from build123d import *

# Parameters (mm, degrees)
F0_R     = 20.6375
F1_DEPTH = 6.35


# Not quite as in the source:
# - a feature names something its author has since deleted; it is built from what else it names


with BuildPart() as f1:
    # F0 (on Top) → F1 (new body)
    with BuildSketch(Plane.XY):
        with BuildLine():
            Line((-44.45, -9.525), (-75.6023437137, -9.525))
            ThreePointArc((-75.6023437137, -9.525), (-65.9911357684, -38.1), (-46.0500638279, -60.7110502417))
            Line((-46.0500638279, -60.7110502417), (-30.473891971, -33.7323291982))
            ThreePointArc((-30.473891971, -33.7323291982), (-17.4625, -30.2459372272), (-13.976108029, -43.2573291982))
            Line((-13.976108029, -43.2573291982), (-29.5522798858, -70.2360502417))
            ThreePointArc((-29.5522798858, -70.2360502417), (0, -76.2), (29.5522798858, -70.2360502417))
            Line((29.5522798858, -70.2360502417), (13.976108029, -43.2573291982))
            ThreePointArc((13.976108029, -43.2573291982), (17.4625, -30.2459372272), (30.473891971, -33.7323291982))
            Line((30.473891971, -33.7323291982), (46.0500638279, -60.7110502417))
            ThreePointArc((46.0500638279, -60.7110502417), (65.9911357684, -38.1), (75.6023437137, -9.525))
            Line((75.6023437137, -9.525), (44.45, -9.525))
            ThreePointArc((44.45, -9.525), (34.925, 0), (44.45, 9.525))
            Line((44.45, 9.525), (75.6023437137, 9.525))
            ThreePointArc((75.6023437137, 9.525), (65.9911357684, 38.1), (46.0500638279, 60.7110502417))
            Line((46.0500638279, 60.7110502417), (30.473891971, 33.7323291982))
            ThreePointArc((30.473891971, 33.7323291982), (17.4625, 30.2459372272), (13.976108029, 43.2573291982))
            Line((13.976108029, 43.2573291982), (29.5522798858, 70.2360502417))
            ThreePointArc((29.5522798858, 70.2360502417), (0, 76.2), (-29.5522798858, 70.2360502417))
            Line((-29.5522798858, 70.2360502417), (-13.976108029, 43.2573291982))
            ThreePointArc((-13.976108029, 43.2573291982), (-17.4625, 30.2459372272), (-30.473891971, 33.7323291982))
            Line((-30.473891971, 33.7323291982), (-46.0500638279, 60.7110502417))
            ThreePointArc((-46.0500638279, 60.7110502417), (-65.9911357684, 38.1), (-75.6023437137, 9.525))
            Line((-75.6023437137, 9.525), (-44.45, 9.525))
            ThreePointArc((-44.45, 9.525), (-34.925, 0), (-44.45, -9.525))
        make_face()
        Circle(F0_R, mode=Mode.SUBTRACT)
    extrude(amount=F1_DEPTH)


solid = f1.part
Geometry: final body of the model. Coordinates: model frame, mm. A direction names the side the tool comes from. Give positions to 0.01 mm unless a question says otherwise; leave off trailing zeros. Loops run counter-clockwise (first coordinate to the right, second up) from the corner with the lowest first, then second, coordinate; pieces in that order, holes last. Notation, with made-up numbers: (-3, -30) - (30, -30) arc R29 cw to (30, 8) - close; hole circle Ø8 at (-29.75, 33.25). An arc over 180 degrees is marked (long way). One line per question, with ' | ' between items. Start each with the question number.
(1) Reachability of faces 1 (the flat face through (38.37, 47.41, 3.13)), 2 (the flat face through (21.655, 56.558, 3.131)), 3 (the flat face through (60, -9.525, 3)), 4 (the flat face through (-60, 9.525, 3)) from +Z, -Z, +X, -X, +Y, -Y: full face, straight path, thin tool, end or side. Return the list, or none.
(2) Section query B-B on x = 0. Return loops of the section in (y, z).
(3) Ray query, line 1 (X direction, y = -55, z = 1.5); line 2 (Y direction, x = 0, z = 4.5); line 3 (X direction, y = -46, z = 4.25). Return the intervals inside material, ascending. Write a range as from..to.
(4) Pull-direction query (X, two-part tool) for faces 5 (the cylindrical face through (-0.4, -76.2, 3.1)), 6 (the flat face through (60, 9.525, 3)), 7 (the flat face through (21.873, -56.936, 3.131)), 8 (the cylindrical face through (65.778, -38.467, 3.131)); classes: released by +X, released by -X, zero draft, split by the parting line, or undercut.
(5) Contact query for flat-ended pins moving along their axis: pin 1 (1 mm diameter, centred on x = -9.5, z = 5, fed in from +Y); pin 2 (1 mm diameter, centred on x = -40.5, z = 1, fed in from +Y); pin 3 (3 mm diameter, centred on x = -63.5, z = 1.5, fed in from +Y). Output: stop coordinate, or through.
(6) Section query D-D on x = 33. Return loops of the section in (y, z).
The answers:
1) face 1: +Z, -Z, +Y | face 2: +Z, -Z | face 3: +Z, -Z, +X | face 4: +Z, -Z, -X
2) outline: (-76.2, 0) - (-20.64, 0) - (-20.64, 6.35) - (-76.2, 6.35) - close; (20.64, 0) - (76.2, 0) - (76.2, 6.35) - (20.64, 6.35) - close
3) line 1: -52.74..-42.75, -20.76..20.76, 42.75..52.74 | line 2: -76.2..-20.64, 20.64..76.2 | line 3: -60.75..-37.56, -15.56..15.56, 37.56..60.75
4) face 5: split by the parting line | face 6: zero draft | face 7: undercut | face 8: released by +X
5) pin 1: y = 75.67 | pin 2: y = 51.96 | pin 3: y = 44.3
6) outline: (-38.11, 0) - (38.11, 0) - (38.11, 6.35) - (-38.11, 6.35) - close
